Design review of the part built by this model. Coordinates are the model's own, in mm. Face numbers are marked on the shaded views. A direction names the side the tool comes from. Coordinates: 2 decimals unless noted, no trailing zeros. Loops run counter-clockwise (first coordinate to the right, second up) from the corner with the lowest first, then second, coordinate; pieces in that order, holes last. Notation, with made-up numbers: M 60,-4.5 L 84,-4.5 A16 ccw 84,13.5 Z; hole C -13.5,-32 d5. An arc over 180 degrees is marked long. One line per item, written item: value.
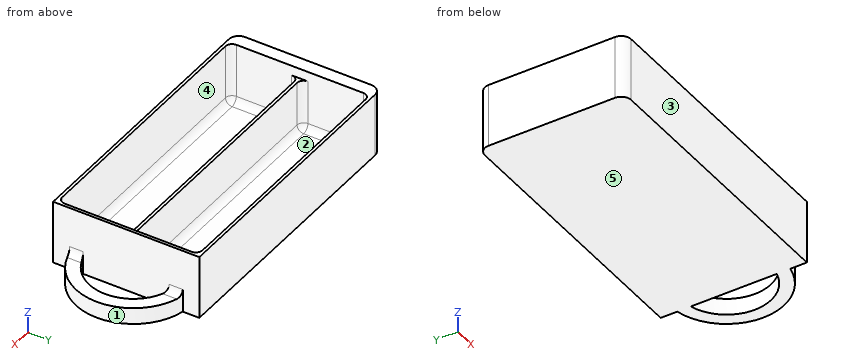
```python
from build123d import *

# Parameters (mm, degrees)
SKETCH_1_W                  = 86
SKETCH_1_H                  = 44.2
EXTRUDE_1_DEPTH             = 14.2
EXTRUDE_2_DEPTH             = 5
SKETCH_3_W                  = 81.1
SKETCH_3_H                  = 42.4
CUT_EXTRUDE_1_DEPTH         = 18.3
HOLE_WIZARD_8_3_8_3_1_D     = 8.3
HOLE_WIZARD_8_3_8_3_1_DEPTH = 3.2
RIB_1_REACH                 = 108.755
SKETCH_6_WALL_W             = 296.60943773
SKETCH_6_WALL_H             = 0.9
FILLET_1_R                  = 3
EXTRUDE_START               = -3.5
SKETCH_7_R                  = 4.15
EXTRUDE_3_DEPTH             = 3.5
FILLET_2_R                  = 2


with BuildPart() as part:
    # Эскиз1 → Бобышка-Вытянуть1 (new body)
    with BuildSketch(Plane.XY.offset(9.6)):
        with Locations((47, 0)):
            Rectangle(SKETCH_1_W, SKETCH_1_H)
    extrude(amount=-EXTRUDE_1_DEPTH)

    # Эскиз2 → Бобышка-Вытянуть2 (add)
    with BuildSketch(Plane(origin=(0, 0, -4.6), x_dir=(-1, 0, 0), z_dir=(0, 0, -1))):
        with BuildLine():
            Line((-90, -22.1), (-90, -17.1))
            ThreePointArc((-90, -17.1), (-104, 0), (-90, 17.1))
            Line((-90, 17.1), (-90, 22.1))
            Line((-90, 22.1), (-4, 22.1))
            Line((-4, 22.1), (-4, -22.1))
            Line((-4, -22.1), (-90, -22.1))
        make_face()
        with BuildLine():
            Line((-90, -12.994779171), (-90, 12.994779171))
            ThreePointArc((-90, 12.994779171), (-100, 0), (-90, -12.994779171))
        make_face(mode=Mode.SUBTRACT)
    extrude(amount=EXTRUDE_2_DEPTH)

    # Эскиз3 → Вырез-Вытянуть1 (cut)
    with BuildSketch(Plane.XY.offset(9.6)):
        with Locations((48.55, 0)):
            Rectangle(SKETCH_3_W, SKETCH_3_H)
    extrude(amount=-CUT_EXTRUDE_1_DEPTH, mode=Mode.SUBTRACT)

    # Диаметр отверстия Ø8.3 (8.3)1
    with Locations(Plane.ZY.offset(-4)):
        with Locations((0, 0)):
            Hole(HOLE_WIZARD_8_3_8_3_1_D / 2, depth=HOLE_WIZARD_8_3_8_3_1_DEPTH)

    # Эскиз6 wall → Ребро1 (add, up to next)
    with BuildSketch(Plane(origin=(48.55, 0, 6.6), x_dir=(1, 0, 0), z_dir=(0, 0, -1)), mode=Mode.PRIVATE) as rib_1_sk1:
        Rectangle(SKETCH_6_WALL_W, SKETCH_6_WALL_H)
    rib_1_tool1 = extrude(rib_1_sk1.sketch, amount=RIB_1_REACH, mode=Mode.PRIVATE) - part.part
    add(rib_1_tool1.solids().sort_by_distance((48.55, 0, 6.6))[0])

    # Скругление1
    fillet_1_edges = [part.edges().sort_by_distance(p)[0] for p in [
        (4, -22.1, 0),
        (4, 22.1, 0),
    ]]
    fillet(fillet_1_edges, radius=FILLET_1_R)

    # Эскиз7 → Бобышка-Вытянуть3 (add)
    with BuildSketch(Plane.ZY.offset(-4).offset(EXTRUDE_START)):
        Circle(SKETCH_7_R)
    extrude(amount=EXTRUDE_3_DEPTH)

    # Скругление2
    fillet_2_edges = [part.edges().sort_by_distance(p)[0] for p in [
        (90, -15.047389586, -4.6),
        (90, 15.047389586, -4.6),
        (8, 10.825, -8.7),
        (8, -21.2, 0.45),
        (48.55, 21.2, -8.7),
        (8, 21.2, 0.45),
        (89.1, -10.825, -8.7),
        (89.1, 21.2, 0.45),
        (48.55, -21.2, -8.7),
        (89.1, -21.2, 0.45),
        (8, -10.825, -8.7),
        (89.1, 10.825, -8.7),
        (48.55, 0.45, -8.7),
        (8, 0.45, -1.05),
        (89.1, 0.45, -1.05),
        (8, -0.45, -1.05),
        (89.1, -0.45, -1.05),
        (48.55, -0.45, -8.7),
    ]]
    fillet(fillet_2_edges, radius=FILLET_2_R)


solid = part.part
```
(1) We need section A-A on z = 8.25. State the section outline as (x, y) points.
Reply:
outline: M 4,-19.1 A3 ccw 7,-22.1 L 90,-22.1 L 90,22.1 L 7,22.1 A3 ccw 4,19.1 Z; hole M 8,-19.2 A2 ccw 10,-21.2 L 87.1,-21.2 A2 ccw 89.1,-19.2 L 89.1,19.2 A2 ccw 87.1,21.2 L 10,21.2 A2 ccw 8,19.2 Z
(2) We need section C-C on x = 48.5. State the section outline as (y, z) points, then the cut area to 3 significant figures.
Reply:
outline: M -22.1,-9.6 L 22.1,-9.6 L 22.1,9.6 L 21.2,9.6 L 21.2,-6.7 A2 cw 19.2,-8.7 L 2.45,-8.7 A2 cw 0.45,-6.7 L 0.45,6.6 L -0.45,6.6 L -0.45,-6.7 A2 cw -2.45,-8.7 L -19.2,-8.7 A2 cw -21.2,-6.7 L -21.2,9.6 L -22.1,9.6 Z
area: 89.9 mm2
(3) Mouldability with a two-part tool opening along Y and no side actions: class the marked faces 1, 2 and 3 as released by +Y, released by -Y, zero draft, split by the parting line, or undercut.
Reply:
face 1: split by the parting line
face 2: undercut
face 3: released by -Y
(4) We need section D-D on z = 1.75. State the section outline as (x, y) points, then the cut area to 3 significant figures.
Reply:
outline: M 4,-19.1 A3 ccw 7,-22.1 L 90,-22.1 L 90,22.1 L 7,22.1 A3 ccw 4,19.1 Z; hole M 8,-19.2 A2 ccw 10,-21.2 L 87.1,-21.2 A2 ccw 89.1,-19.2 L 89.1,-2.45 A2 ccw 87.1,-0.45 L 10,-0.45 A2 ccw 8,-2.45 Z; hole M 8,2.45 A2 ccw 10,0.45 L 87.1,0.45 A2 ccw 89.1,2.45 L 89.1,19.2 A2 ccw 87.1,21.2 L 10,21.2 A2 ccw 8,19.2 Z
area: 439 mm2
(5) Tool access review of the marked faces 4 and 5: name each direction out of +Z, -Z, +X, -X, +Y, -Y from which nothing blocks a thin tool from reaching the whole face with its end or side.
Reply:
face 4: +Z
face 5: -Z, +X, -X, +Y, -Y
(6) To check wall thickness, follow line 1 along Y through (x, z) = (74, 0.75); line 2 along X through (y, z) = (8.5, 0.5); line 3 along Y through (x, z) = (18, 8.75). State the ranges of each line that lie inside material, in increasing order. Write a range as [from, to].
Reply:
line 1: y = [-22.1, -21.2], [-0.45, 0.45], [21.2, 22.1]
line 2: x = [4, 8], [89.1, 90]
line 3: y = [-22.1, -21.2], [21.2, 22.1]
(7) We need section B-B on y = 11. State the section outline as (x, z) points.
Reply:
outline: M 4,-9.6 L 90,-9.6 L 90,9.6 L 89.1,9.6 L 89.1,-6.7 A2 cw 87.1,-8.7 L 10,-8.7 A2 cw 8,-6.7 L 8,9.6 L 4,9.6 Z; M 94.28,-9.6 L 100.09,-9.6 L 100.09,-4.6 L 94.28,-4.6 Z
(8) Insertion check: pin 1 (13.5 mm diameter, centred on x = 36.5, y = 14, fed in from +Z); pin 2 (5.5 mm diameter, centred on x = 54, y = -1, fed in from +Z); pin 3 (1.5 mm diameter, centred on y = 8.5, z = 6.5, fed in from +X). Each pin has a flat end and moves straight along its axis. Give the tip position at first contact, or say it passes through.
Reply:
pin 1: stops at z = -7.96
pin 2: stops at z = 6.6
pin 3: stops at x = 90
